from build123d import *

# Parameters (mm, degrees)
SKETCH2_W           = 48
SKETCH2_H           = 80
BOSS_EXTRUDE1_DEPTH = 0.5
SKETCH3_W           = 48
SKETCH3_H           = 1
BOSS_EXTRUDE2_DEPTH = 2.5
SKETCH4_W           = 1.9
SKETCH4_H           = 0.4
BOSS_EXTRUDE3_DEPTH = 0.8
SKETCH5_W           = 1.9
SKETCH5_H           = 0.4
BOSS_EXTRUDE4_DEPTH = 0.8
SKETCH6_R           = 4.1
CUT_EXTRUDE2_DEPTH  = 0.5


with BuildPart() as part:
    # Sketch2 → Boss-Extrude1 (new body)
    with BuildSketch(Plane.XY):
        with Locations((24, 40)):
            Rectangle(SKETCH2_W, SKETCH2_H)
    extrude(amount=BOSS_EXTRUDE1_DEPTH)

    # Sketch3 → Boss-Extrude2 (add)
    with BuildSketch(Plane.XY.offset(0.5)):
        with Locations((24, 79.5)):
            Rectangle(SKETCH3_W, SKETCH3_H)
        with Locations((24, 0.5)):
            Rectangle(SKETCH3_W, SKETCH3_H)
    extrude(amount=BOSS_EXTRUDE2_DEPTH)

    # Sketch4 → Boss-Extrude3 (add)
    with BuildSketch(Plane.XY.offset(3)):
        with Locations((6.05, 79.5)):
            Rectangle(SKETCH4_W, SKETCH4_H)
        with Locations((41.95, 79.5)):
            Rectangle(SKETCH4_W, SKETCH4_H)
    extrude(amount=BOSS_EXTRUDE3_DEPTH)

    # Sketch5 → Boss-Extrude4 (add)
    with BuildSketch(Plane.XY.offset(3)):
        with Locations((6.05, 0.5)):
            Rectangle(SKETCH5_W, SKETCH5_H)
        with Locations((41.95, 0.5)):
            Rectangle(SKETCH5_W, SKETCH5_H)
    extrude(amount=BOSS_EXTRUDE4_DEPTH)

    # Sketch6 → Cut-Extrude2 (cut)
    with BuildSketch(Plane(origin=(0, 0, 0), x_dir=(-1, 0, 0), z_dir=(0, 0, -1))):
        with Locations((-24, 40)):
            Circle(SKETCH6_R)
    extrude(amount=-CUT_EXTRUDE2_DEPTH, mode=Mode.SUBTRACT)


solid = part.part
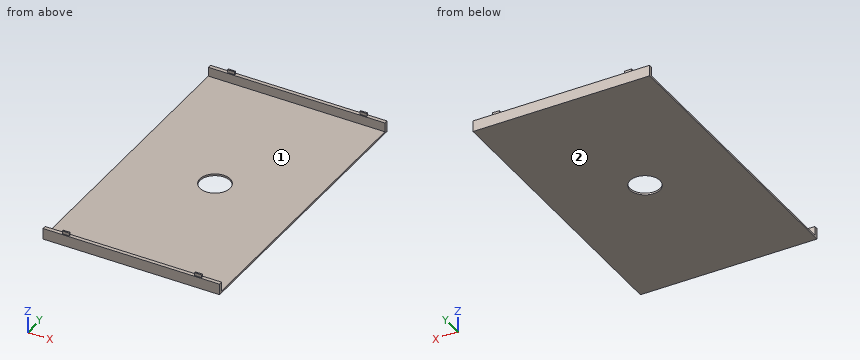
The listing builds one solid part. Answer for the finished solid, in the listing's coordinates (mm). Face numbers are marked on the shaded views. Give positions to 0.01 mm unless a question says otherwise; leave off trailing zeros. Write each loop counter-clockwise with the first axis right and the second up, starting at its lowest first coordinate (ties: lowest second). Pieces come first, ordered by that corner, then holes. Notation, with made-up numbers: (87, 76.25) - (105, 76.25) arc R3 cw to (105, 81.25) - close; hole circle Ø5 at (73, 8). An arc over 180 degrees is marked (long way). Use a Markdown table: item, result.
1. Section C-C on z = 2.2 is taken. Write down the section's boundary in (x, y), plus the area to 3 significant figures.
Values follow:
| item | result |
|---|---|
| outline | (0, 0) - (48, 0) - (48, 1) - (0, 1) - close; (0, 79) - (48, 79) - (48, 80) - (0, 80) - close |
| area | 96.0 mm² |
2. For a pull along Y with two mould halves and no side action, classify the marked faces 1 and 2 as released by +Y, released by -Y, zero draft, split by the parting line, or undercut.
Values follow:
| item | result |
|---|---|
| face 1 | undercut |
| face 2 | zero draft |
3. Section A-A on y = 40 is taken. Write down the section's boundary in (x, z).
Values follow:
| item | result |
|---|---|
| outline | (0, 0) - (19.9, 0) - (19.9, 0.5) - (0, 0.5) - close; (28.1, 0) - (48, 0) - (48, 0.5) - (28.1, 0.5) - close |
4. Section D-D on x = 6 is taken. Write down the section's boundary in (y, z), plus the area to 3 significant figures.
Values follow:
| item | result |
|---|---|
| outline | (0, 0) - (80, 0) - (80, 3) - (79.7, 3) - (79.7, 3.8) - (79.3, 3.8) - (79.3, 3) - (79, 3) - (79, 0.5) - (1, 0.5) - (1, 3) - (0.7, 3) - (0.7, 3.8) - (0.3, 3.8) - (0.3, 3) - (0, 3) - close |
| area | 45.6 mm² |
5. Section B-B on x = 24 is taken. Write down the section's boundary in (y, z), plus the area to 3 significant figures.
Values follow:
| item | result |
|---|---|
| outline | (0, 0) - (35.9, 0) - (35.9, 0.5) - (1, 0.5) - (1, 3) - (0, 3) - close; (44.1, 0) - (80, 0) - (80, 3) - (79, 3) - (79, 0.5) - (44.1, 0.5) - close |
| area | 40.9 mm² |
6. Each of these flat-tipped pins is pushed along its axis until it touches: P1, Ø1, axis at x = 14.5, y = 39, coming from the +Z side; P2, Ø0.9, axis at x = 6, z = 3.5, coming from the +Y side; P3, Ø0.6, axis at x = 5.5, z = 3.5, coming from the -Y side. Where does it stop, or does it pass through?
Values follow:
| item | result |
|---|---|
| P1 | stops at z = 0.5 |
| P2 | stops at y = 79.7 |
| P3 | stops at y = 0.3 |
7. Find the intervals of material crossed by probe 1 along Y at (x, z) = (29.5, 1.1); probe 2 along Y at (x, z) = (24, 0.25); probe 3 along Z at (x, y) = (15.5, 43.5), in increasing order. Write a range as from..to.
Values follow:
| item | result |
|---|---|
| probe 1 | y = 0..1, 79..80 |
| probe 2 | y = 0..35.9, 44.1..80 |
| probe 3 | z = 0..0.5 |
